Model file for the job. Use its own axes, mm. A direction names the side the tool comes from. Coordinates: 2 decimals unless noted, no trailing zeros. Write each loop counter-clockwise with the first axis right and the second up, starting at its lowest first coordinate (ties: lowest second). Pieces come first, ordered by that corner, then holes.
Q1. Pull direction Y, two halves, no side cores. Call faces 1 (the flat face through (0, -8, 0)), 2 (the flat face through (0, 0, -59.62)), 3 (the flat face through (0, 0, -58.62)), 4 (the cylindrical face through (-4.09, -18.43, -35.67)): released by +Y, released by -Y, zero draft, split by the parting line, or undercut.
Q2. Band-saw the part on A-A, the plane z = 6.5. Write the cut outline in (x, y) (3 decimals).
Q3. Pin check, flat tips, straight feed: P1, Ø4, axis at x = 7.5, z = -15, coming from the +Y side; P2, Ø1.5, axis at x = 9.5, z = -51, coming from the -Y side; P3, Ø6, axis at y = -4.5, z = -31.5, coming from the +X side; P4, Ø20.5, axis at x = 1, y = 3.5, coming from the +Z side. Stop position of each tip, or through.
Q4. Drill centre lines: probe 1 along Y at (x, z) = (0, -1.7) (3 decimals); probe 2 along Y at (x, z) = (0, -36.5); probe 3 along Z at (x, y) = (1, 5). Where is each one in solid material? Low to high.
Q5. Which spindle directions (+Z, -Z, +X, -X, +Y, -Y) get a long thin tool onto all of the face, cutting with end or side? Do faces 5 (the cylindrical face through (4.09, -7.87, 7.48)), 6 (the cylindrical face through (-17.813, 0.784, -34.463)), 7 (the flat face through (0, -8, 14.63)). Say none if no direction does.
Q6. Band-saw the part on B-B, the plane z = -33.5. Write the cut outline in (x, y).
from build123d import *

# Parameters (mm, degrees)
SKETCH2_R           = 8.87
SKETCH2_R_2         = 7.825
BOSS_EXTRUDE1_DEPTH = 14.63
SKETCH3_R           = 11.735
SKETCH3_R_2         = 10.685
BOSS_EXTRUDE2_DEPTH = 2.63
FILLET1_R           = 2.5
FILLET2_R           = 1
SKETCH6_R           = 7.825
CUT_EXTRUDE2_DEPTH  = 18.63
SKETCH7_R           = 18.88
BOSS_EXTRUDE3_DEPTH = 1
SKETCH10_R          = 18.88
SKETCH10_R_2        = 17.83
BOSS_EXTRUDE4_DEPTH = 49
FILLET3_R           = 2.5
FILLET6_R           = 10


# Read off the part's stored shape, not the designer's step: Loft5, Loft6
with BuildPart() as part:
    # Sketch2 → Boss-Extrude1 (new body)
    with BuildSketch(Plane.XY):
        Circle(SKETCH2_R)
        Circle(SKETCH2_R_2, mode=Mode.SUBTRACT)
    extrude(amount=BOSS_EXTRUDE1_DEPTH)


with BuildPart() as body_2:
    # Sketch3 → Boss-Extrude2 (new body)
    with BuildSketch(Plane(origin=(0, 0, -2.1), x_dir=(-1, 0, 0), z_dir=(0, 0, -1))):
        Circle(SKETCH3_R)
        Circle(SKETCH3_R_2, mode=Mode.SUBTRACT)
    extrude(amount=-BOSS_EXTRUDE2_DEPTH)


    add(part.part)  # loft1 joins it to this body
    # loft up to a face of the part (loft1)
    loft([Face(Wire([body_2.edges().sort_by_distance((8.033160288, -8.554446843, 0.53))[0]])), Face(Wire([body_2.edges().sort_by_distance((-6.07193283, -6.465951725, 0))[0]]))])

    # Fillet1
    fillet1_edges = [body_2.edges().sort_by_distance(p)[0] for p in [
        (11.735, 0, 0.53),
    ]]
    fillet(fillet1_edges, radius=FILLET1_R)

    # Fillet2
    fillet2_edges = [body_2.edges().sort_by_distance(p)[0] for p in [
        (10.685, 0, 0.335759162),
    ]]
    fillet(fillet2_edges, radius=FILLET2_R)

    # Sketch6 → Cut-Extrude2 (cut)
    with BuildSketch(Plane.XY.offset(14.63)):
        Circle(SKETCH6_R)
    extrude(amount=-CUT_EXTRUDE2_DEPTH, mode=Mode.SUBTRACT)



with BuildPart() as body_2_2:
    # Sketch7 → Boss-Extrude3 (new body)
    with BuildSketch(Plane.XY.offset(-59.62)):
        Circle(SKETCH7_R)
    extrude(amount=BOSS_EXTRUDE3_DEPTH)

    # Sketch10 → Boss-Extrude4 (add)
    with BuildSketch(Plane.XY.offset(-58.62)):
        Circle(SKETCH10_R)
        Circle(SKETCH10_R_2, mode=Mode.SUBTRACT)
    extrude(amount=BOSS_EXTRUDE4_DEPTH)

    # Fillet3
    fillet3_edges = [body_2_2.edges().sort_by_distance(p)[0] for p in [
        (-18.88, 0, -59.62),
    ]]
    fillet(fillet3_edges, radius=FILLET3_R)


with BuildPart() as body_3:
    # Loft5 outline → Loft5 (revolve)
    with BuildSketch(Plane.XZ):
        Polygon((10.685, -2.1), (0, -2.1), (0, -9.62), (17.83, -9.62), align=None)
    revolve(axis=Axis((0, 0, 0), (0, 0, 1)))


with BuildPart() as body_2_1:
    add(body_2.part)

    add(body_2_2.part)  # Loft6 merges body 2 2

    add(body_3.part)  # Loft6 merges body 3
    # Loft6 outline → Loft6 (revolve)
    with BuildSketch(Plane.XZ):
        Polygon((18.88, -9.62), (11.735, -2.1), (10.685, -2.1), (17.83, -9.62), align=None)
    revolve(axis=Axis((0, 0, 0), (0, 0, 1)))

    # Fillet6
    fillet6_edges = [body_2_1.edges().sort_by_distance(p)[0] for p in [
        (-18.88, 0, -9.62),
    ]]
    fillet(fillet6_edges, radius=FILLET6_R)


solid = body_2_1.part
Answer sheet:
1. face 1: undercut
1. face 2: zero draft
1. face 3: undercut
1. face 4: split by the parting line
2. outline: circle Ø17.74 at (0, 0); hole circle Ø15.65 at (0, 0)
3. P1: stops at y = 18.06
3. P2: stops at y = -16.73
3. P3: stops at x = 18.82
3. P4: stops at z = 14.63
4. probe 1: y = -11.72 to -10.685, 10.685 to 11.72
4. probe 2: y = -18.88 to -17.83, 17.83 to 18.88
4. probe 3: z = -59.62 to -58.62, -9.62 to -2.1
5. face 5: +Z
5. face 6: none
5. face 7: +Z, +X, -X, +Y, -Y
6. outline: circle Ø37.76 at (0, 0); hole circle Ø35.66 at (0, 0)
